Geometry check sheet. Reference: the model listing, model coordinates, mm. A direction names the side the tool comes from. Round coordinates to 2 decimals unless told otherwise and drop trailing zeros. Write each loop counter-clockwise with the first axis right and the second up, starting at its lowest first coordinate (ties: lowest second). Pieces come first, ordered by that corner, then holes.
Item 1: Cross-section at C-C (x = 428). Enter the section's corners in (y, z) (3 decimals).
Item 2: Scan lines: probe 1 along Z at (x, y) = (292.1, 2.5) (3 decimals); probe 2 along Z at (x, y) = (93, 2) (3 decimals); probe 3 along Z at (x, y) = (108.5, 3.75) (3 decimals). Record each from-to range of solid material in increasing order.
Item 3: Cross-section at A-A (x = 45.5). Enter the section's corners in (y, z) (3 decimals), then the cut area to 3 significant figures.
Item 4: Cross-section at B-B (y = 1.75). State how many separate pieces and enclosed holes the cut face has, then the cut area to 3 significant figures.
Item 5: Depth check by flat-ended pin: P1, Ø3, axis at y = 3, z = -16.5, coming from the -X side; P2, Ø3, axis at x = 568.325, z = -3.175, coming from the +Y side. Enter the tip coordinate at first touch or a pass-through.
Item 6: Access from +Z, -Z, +X, -X, +Y, -Y to the whole of each face (thin tool, end or side, straight path). Record for faces 1 (the face through (551.62, 3.22, -19.11)), 2 (the face through (285, 6.35, -25)).
Item 7: Draft check along X on faces 3 (the face through (285, 0, -25)), 4 (the face through (564.7, 3.1, -19.5)), 5 (the face through (430.881, 3.219, -19.787)). Enter one of: pulls with the +X half, pulls with the -X half, needs draft (parallel to the pull), parting line crosses it, or undercut.
from build123d import *

# Parameters (mm, degrees)
BOSS_EXTRUDE1_DEPTH       = 6.35
FILLET1_R                 = 6.35
CUT_EXTRUDE1_DEPTH        = 6.35
FILLET2_R                 = 2.54
F_6_CLEARANCE_HOLE1_D     = 3.7973
F_6_CLEARANCE_HOLE1_DEPTH = 12.7
F_6_CLEARANCE_HOLE1_TIP   = 1.140824014


with BuildPart() as part:
    # Sketch1 → Boss-Extrude1 (new body)
    with BuildSketch(Plane(origin=(0, 0, 0), x_dir=(1, 0, 0), z_dir=(0, 1, 0))):
        Polygon((0, 0), (577.85, 0), (577.85, 6.35), (549.275, 34.925), (28.575, 34.925), (0, 6.35), align=None)
    extrude(amount=BOSS_EXTRUDE1_DEPTH)

    # Fillet1
    fillet1_edges = [part.edges().sort_by_distance(p)[0] for p in [
        (549.275, 3.175, -34.925),
        (28.575, 3.175, -34.925),
    ]]
    fillet(fillet1_edges, radius=FILLET1_R)

    # Sketch2 → Cut-Extrude1 (cut)
    with BuildSketch(Plane(origin=(0, 6.35, 0), x_dir=(1, 0, 0), z_dir=(0, 1, 0))):
        Polygon((16.645384182, 9.525), (71.415498994, 9.525), (32.520384182, 25.4), align=None)
        Polygon((57.726423324, 25.4), (96.621538136, 9.525), (135.516652948, 25.4), align=None)
        Polygon((121.827577279, 9.525), (160.722692091, 25.4), (199.617806903, 9.525), align=None)
        Polygon((185.928731233, 25.4), (224.823846045, 9.525), (263.718960858, 25.4), align=None)
        Polygon((250.029885188, 9.525), (288.925, 25.4), (327.820114812, 9.525), align=None)
        Polygon((314.131039142, 25.4), (353.026153955, 9.525), (391.921268767, 25.4), align=None)
        Polygon((378.232193097, 9.525), (417.127307909, 25.4), (456.022422721, 9.525), align=None)
        Polygon((442.333347052, 25.4), (481.228461864, 9.525), (520.123576676, 25.4), align=None)
        Polygon((561.204615818, 9.525), (506.434501006, 9.525), (545.329615818, 25.4), align=None)
    extrude(amount=-CUT_EXTRUDE1_DEPTH, mode=Mode.SUBTRACT)

    # Fillet2
    fillet2_edges = [part.edges().sort_by_distance(p)[0] for p in [
        (32.520384182, 3.175, -25.4),
        (71.415498994, 3.175, -9.525),
        (185.928731233, 3.175, -25.4),
        (263.718960858, 3.175, -25.4),
        (224.823846045, 3.175, -9.525),
        (327.820114812, 3.175, -9.525),
        (250.029885188, 3.175, -9.525),
        (288.925, 3.175, -25.4),
        (57.726423324, 3.175, -25.4),
        (135.516652948, 3.175, -25.4),
        (96.621538136, 3.175, -9.525),
        (199.617806903, 3.175, -9.525),
        (121.827577279, 3.175, -9.525),
        (160.722692091, 3.175, -25.4),
        (442.333347052, 3.175, -25.4),
        (520.123576676, 3.175, -25.4),
        (481.228461864, 3.175, -9.525),
        (506.434501006, 3.175, -9.525),
        (545.329615818, 3.175, -25.4),
        (561.204615818, 3.175, -9.525),
        (314.131039142, 3.175, -25.4),
        (391.921268767, 3.175, -25.4),
        (353.026153955, 3.175, -9.525),
        (456.022422721, 3.175, -9.525),
        (378.232193097, 3.175, -9.525),
        (417.127307909, 3.175, -25.4),
        (16.645384182, 3.175, -9.525),
    ]]
    fillet(fillet2_edges, radius=FILLET2_R)

    # 6 Clearance Hole1
    with Locations(Plane(origin=(0, 6.35, 0), x_dir=(1, 0, 0), z_dir=(0, 1, 0))):
        with Locations((12.7, 3.175), (76.2, 3.175), (292.1, 3.175), (568.325, 3.175), (498.475, 3.175)):
            Hole(F_6_CLEARANCE_HOLE1_D / 2, depth=F_6_CLEARANCE_HOLE1_DEPTH)
            with Locations((0, 0, -(F_6_CLEARANCE_HOLE1_DEPTH + F_6_CLEARANCE_HOLE1_TIP / 2))):  # 118° drill point
                Cone(0, F_6_CLEARANCE_HOLE1_D / 2, F_6_CLEARANCE_HOLE1_TIP, mode=Mode.SUBTRACT)


solid = part.part
Resolved:
1. outline: (0, -34.925) - (6.35, -34.925) - (6.35, -20.962) - (0, -20.962) - close; (0, -9.525) - (6.35, -9.525) - (6.35, 0) - (0, 0) - close
2. probe 1: z = -34.925 to -24.104, -9.525 to -5.074, -1.276 to 0
2. probe 2: z = -34.925 to -25.4, -11.003 to 0
2. probe 3: z = -34.925 to -25.4, -14.373 to 0
3. outline: (0, -34.925) - (6.35, -34.925) - (6.35, -20.102) - (0, -20.102) - close; (0, -9.525) - (6.35, -9.525) - (6.35, 0) - (0, 0) - close
3. area: 155 mm2
4. separate pieces: 1
4. enclosed holes: 14
4. area: 14,500 mm2
5. P1: stops at x = 8.65
5. P2: passes through
6. face 1: +Y, -Y
6. face 2: +Z, -Z, +X, -X, +Y
7. face 3: needs draft
7. face 4: pulls with the +X half
7. face 5: undercut
